Here's the drawing with two shaded views (mm, measured from the low corner). I have some questions. Round coordinates to 2 decimals unless told otherwise and drop trailing zeros. Order: outer loops, then holes, each group sorted by start corner. A loop starts at its lowest first (then second) coordinate and runs counter-clockwise, first axis right, second up. Notation, with made-up numbers: (-37, 33) - (-24, 33) arc R26 cw to (-24, 64) - close; hole circle Ø3 at (23, -19.75). An arc over 180 degrees is marked (long way). One line per item, written item: value.
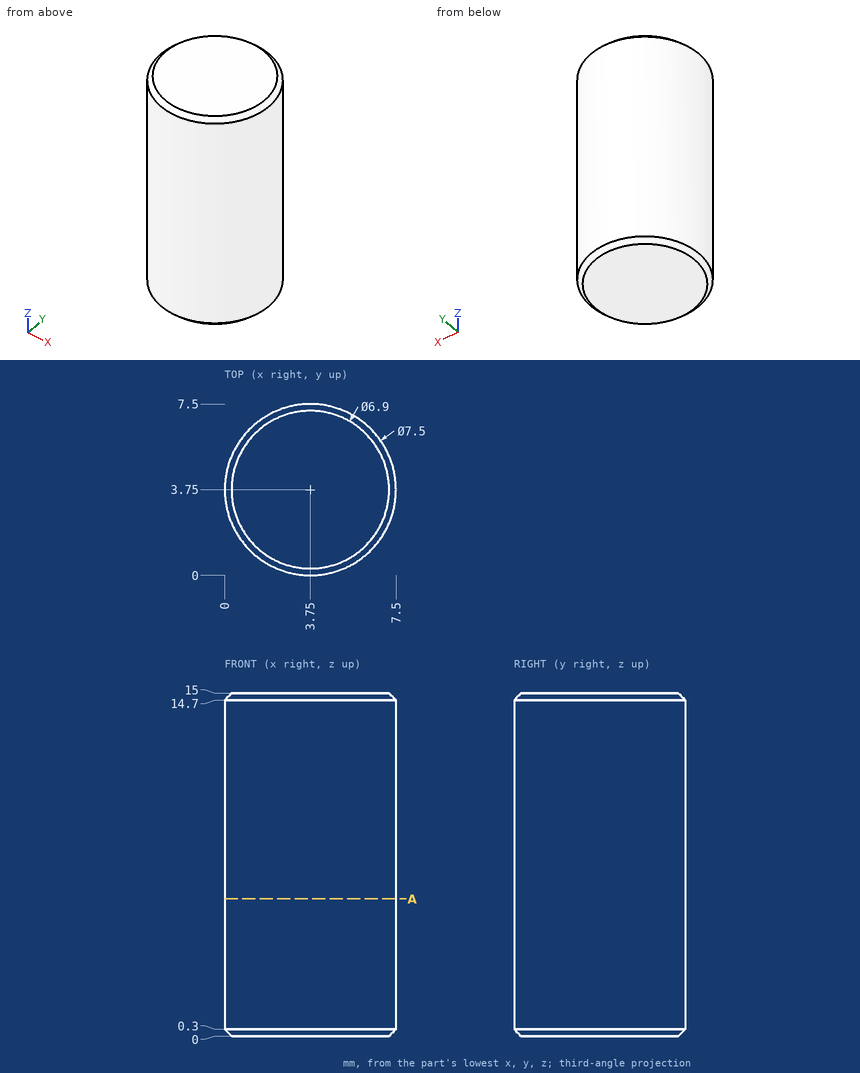
Q1. If we section it at A-A, the plane z = 6: Please give me the cut outline in (x, y).
Results list:
outline: circle Ø7.5 at (3.75, 3.75)
Q2. If I drill on line 1 along X through (y, z) = (5, 12); line 2 along Y through (x, z) = (3.25, 7), over which ranges is the centre line in solid material (lowest first)?
Results list:
line 1: 0.21 to 7.29
line 2: 0.03 to 7.47
Q3. Will these pins go through, and if not, where does the flat tip stop? pin 1 (3 mm diameter, centred on y = 6, z = 6.5, fed in from -X); pin 2 (4 mm diameter, centred on x = 6, z = 8.5, fed in from -Y).
Results list:
pin 1: x = 0.08
pin 2: y = 0.01
